The drawing under review shows one solid part. Ordinate dimensions are in mm from its lowest x, y, z. Coordinates: 2 decimals unless noted, no trailing zeros. Write each loop counter-clockwise with the first axis right and the second up, starting at its lowest first coordinate (ties: lowest second). Pieces come first, ordered by that corner, then holes. Notation, with made-up numbers: M -16,60.5 L 41,60.5 A32 cw 41,95.5 Z; hole C -39.75,-9 d2. An arc over 180 degrees is marked long. Answer as CSV lines item,"result". Start each with the question number.
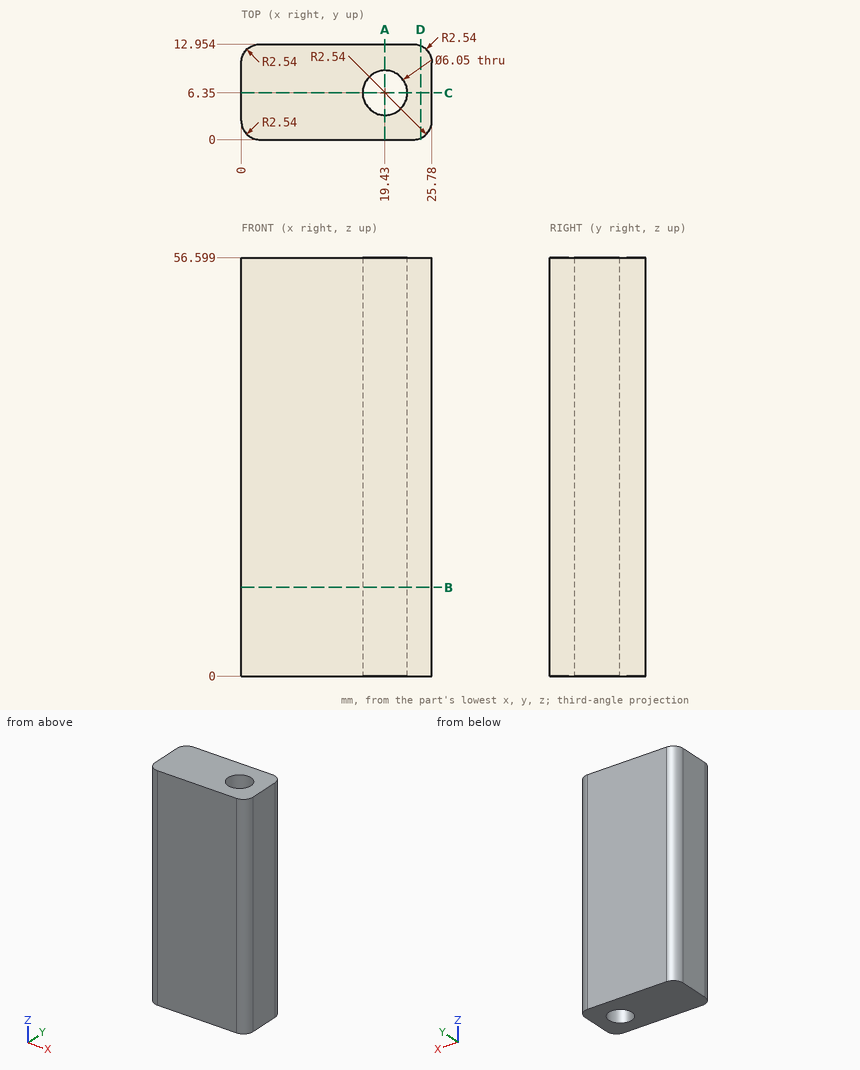
1) Take a section at D-D on x = 24.25. Give the boundary of the cut face in (y, z).
2) Take a section at B-B on z = 12. Give the boundary of the cut face in (x, y) (3 decimals).
3) To check wall thickness, follow line 1 (Y direction, x = 19.43, z = 38.5) (3 decimals); line 2 (X direction, y = 6, z = 22) (1 decimal); line 3 (X direction, y = 4.5, z = 35.5). State the ranges of each line that lie inside material, in increasing order. Write a range as [from, to].
4) Take a section at C-C on y = 6.35. Give the boundary of the cut face in (x, z) (1 decimal), and give its area (3 significant figures).
5) Take a section at A-A on x = 19.43. Give the boundary of the cut face in (y, z) (1 decimal).
Results:
1,outline,"M 0.21,0 L 12.74,0 L 12.74,56.6 L 0.21,56.6 Z"
2,outline,"M 0,2.54 A2.54 ccw 2.54,0 L 23.24,0 A2.54 ccw 25.78,2.54 L 25.78,10.414 A2.54 ccw 23.24,12.954 L 2.54,12.954 A2.54 ccw 0,10.414 Z; hole C 19.43,6.35 d6.05"
3,line 1,"y = [0, 3.325], [9.375, 12.954]"
3,line 2,"x = [0, 16.4], [22.4, 25.8]"
3,line 3,"x = [0, 17.04], [21.82, 25.78]"
4,outline,"M 0,0 L 16.4,0 L 16.4,56.6 L 0,56.6 Z; M 22.5,0 L 25.8,0 L 25.8,56.6 L 22.5,56.6 Z"
4,area,"1,120 mm²"
5,outline,"M 0,0 L 3.3,0 L 3.3,56.6 L 0,56.6 Z; M 9.4,0 L 13,0 L 13,56.6 L 9.4,56.6 Z"
